Could you check a few things on this model? Use its own coordinates, in mm. Round coordinates to 2 decimals unless told otherwise and drop trailing zeros. Loops run counter-clockwise (first coordinate to the right, second up) from the corner with the lowest first, then second, coordinate; pieces in that order, holes last. Notation, with made-up numbers: M 20,30 L 75,30 A29 cw 75,52 Z; hole C 84.5,1 d1. An arc over 180 degrees is marked long. One line per item, written item: value. Start each with the question number.
Q1. Imagine slicing it at B-B (x = 77). Please give me the cut outline in (y, z), then the cut area to 3 significant figures.
Q2. Imagine slicing it at A-A (y = -88). Please give me the cut outline in (x, z).
Q3. Thinking about a two-plate mould opening in X: for faces 1 (the face through (-70.457, -91.67, 2.465)), 2 (the face through (-2, 2, 5)), which applies, released by +X, released by -X, zero draft, split by the parting line, or undercut?
Q4. Imagine slicing it at C-C (z = 2.85). Give the number of separate pieces and of enclosed holes in the cut face, then the cut area to 3 significant figures.
Q5. Please list where these lines run through material, in increasing order: line 1 along Y through (x, z) = (125.5, 3.5); line 2 along X through (y, z) = (-76.5, 0.7); line 3 along X through (y, z) = (-87, 2.8).
from build123d import *

# Parameters (mm, degrees)
ESQUISSE1_W             = 300
ESQUISSE1_H             = 300
BOSS_EXTRU_1_DEPTH      = 5
ENL_V_MAT_EXTRU_1_DEPTH = 5
CONG_1_R                = 5


with BuildPart() as part:
    # Esquisse1 → Boss.-Extru.1 (new body)
    with BuildSketch(Plane.XY):
        Rectangle(ESQUISSE1_W, ESQUISSE1_H)
    extrude(amount=BOSS_EXTRU_1_DEPTH)

    # Esquisse2 → Enlèv. mat.-Extru.1 (cut)
    with BuildSketch(Plane.XY):
        Polygon((-70.753787975, 49.54058454), (-49.54058454, 70.753787975), (-91.966991411, 113.180194847), (-81.360389693, 123.786796564), (-102.573593129, 145), (-145, 102.573593129), (-123.786796564, 81.360389693), (-113.180194847, 91.966991411), align=None)
        Polygon((145, 102.573593129), (123.786796564, 81.360389693), (113.180194847, 91.966991411), (70.753787975, 49.54058454), (49.54058454, 70.753787975), (91.966991411, 113.180194847), (81.360389693, 123.786796564), (102.573593129, 145), align=None)
        Polygon((-70.753787975, -49.54058454), (-49.54058454, -70.753787975), (-91.966991411, -113.180194847), (-81.360389693, -123.786796564), (-102.573593129, -145), (-145, -102.573593129), (-123.786796564, -81.360389693), (-113.180194847, -91.966991411), align=None)
        Polygon((91.966991411, -113.180194847), (81.360389693, -123.786796564), (102.573593129, -145), (145, -102.573593129), (123.786796564, -81.360389693), (113.180194847, -91.966991411), (70.753787975, -49.54058454), (49.54058454, -70.753787975), align=None)
    extrude(amount=ENL_V_MAT_EXTRU_1_DEPTH, mode=Mode.SUBTRACT)

    # Congé1
    cong_1_edges = [part.edges().sort_by_distance(p)[0] for p in [
        (-150, 150, 2.5),
        (150, 150, 2.5),
        (150, -150, 2.5),
        (-150, -150, 2.5),
    ]]
    fillet(cong_1_edges, radius=CONG_1_R)


solid = part.part
Report:
1. outline: M -150,0 L -98.21,0 L -98.21,5 L -150,5 Z; M -55.79,0 L 55.79,0 L 55.79,5 L -55.79,5 Z; M 98.21,0 L 150,0 L 150,5 L 98.21,5 Z
1. area: 1,080 mm²
2. outline: M -150,0 L -130.43,0 L -130.43,5 L -150,5 Z; M -117.15,0 L -109.21,0 L -109.21,5 L -117.15,5 Z; M -66.79,0 L 66.79,0 L 66.79,5 L -66.79,5 Z; M 109.21,0 L 117.15,0 L 117.15,5 L 109.21,5 Z; M 130.43,0 L 150,0 L 150,5 L 130.43,5 Z
3. face 1: undercut
3. face 2: zero draft
4. separate pieces: 1
4. enclosed holes: 4
4. area: 75,600 mm²
5. line 1: y = -150 to -122.07, -83.07 to 83.07, 122.07 to 150
5. line 2: x = -150 to -97.71, -55.29 to 55.29, 97.71 to 150
5. line 3: x = -150 to -129.43, -118.15 to -108.21, -65.79 to 65.79, 108.21 to 118.15, 129.43 to 150
